Read the model definition and answer for the solid it produces. Units are mm, in the model's axes. Face numbers are marked on the shaded views. A direction names the side the tool comes from. Coordinates: 2 decimals unless noted, no trailing zeros. Write each loop counter-clockwise with the first axis right and the second up, starting at its lowest first coordinate (ties: lowest second). Pieces come first, ordered by that corner, then holes. Notation, with made-up numbers: M 69.5,-38 L 115.5,-38 A20 ccw 115.5,-24 Z; hole C 77,-37.75 d10. An arc over 180 degrees is marked long. Write item = value, one per line.
from build123d import *

# Parameters (mm, degrees)
BOSS_EXTRUDE1_DEPTH = 20
SKETCH7_R           = 70
CUT_EXTRUDE1_DEPTH  = 149.354929298


with BuildPart() as part:
    # Sketch4 → Boss-Extrude1 (new body)
    with BuildSketch(Plane.XY):
        Polygon((-50, -86.602540378), (50, -86.602540378), (100, 0), (50, 86.602540378), (-50, 86.602540378), (-100, 0), align=None)
        Polygon((-50, -86.602540378), (-110, 0), (-100, 0), align=None)
        Polygon((-100, 0), (-55, 95.262794416), (-50, 86.602540378), align=None)
        Polygon((-50, 86.602540378), (55, 95.262794416), (50, 86.602540378), align=None)
        Polygon((50, 86.602540378), (110, 0), (100, 0), align=None)
        Polygon((100, 0), (55, -95.262794416), (50, -86.602540378), align=None)
        Polygon((50, -86.602540378), (-55, -95.262794416), (-50, -86.602540378), align=None)
        with BuildLine():
            Line((-55, 95.262794416), (-50, 86.602540378))
            Line((-50, 86.602540378), (-50.900048654, 97.515050362))
            ThreePointArc((-50.900048654, 97.515050362), (-52.961998078, 96.410719111), (-55, 95.262794416))
        make_face()
        with BuildLine():
            Line((55, 95.262794416), (50, 86.602540378))
            Line((50, 86.602540378), (59.000486538, 92.838260369))
            ThreePointArc((59.000486538, 92.838260369), (57.013132909, 94.071795327), (55, 95.262794416))
        make_face()
        with BuildLine():
            Line((110, 0), (100, 0))
            Line((100, 0), (109.900535191, -4.676789993))
            ThreePointArc((109.900535191, -4.676789993), (109.975130987, -2.338923785), (110, 0))
        make_face()
        with BuildLine():
            Line((55, -95.262794416), (50, -86.602540378))
            Line((50, -86.602540378), (50.900048654, -97.515050362))
            ThreePointArc((50.900048654, -97.515050362), (52.961998078, -96.410719111), (55, -95.262794416))
        make_face()
        with BuildLine():
            Line((-55, -95.262794416), (-50, -86.602540378))
            Line((-50, -86.602540378), (-59.000486538, -92.838260369))
            ThreePointArc((-59.000486538, -92.838260369), (-57.013132909, -94.071795327), (-55, -95.262794416))
        make_face()
        with BuildLine():
            Line((-110, 0), (-100, 0))
            Line((-100, 0), (-109.900535191, 4.676789993))
            ThreePointArc((-109.900535191, 4.676789993), (-109.975130987, 2.338923785), (-110, 0))
        make_face()
    extrude(amount=BOSS_EXTRUDE1_DEPTH)

    # Sketch7 → Cut-Extrude1 (cut, through all)
    with BuildSketch(Plane(origin=(0, 0, 0), x_dir=(-1, 0, 0), z_dir=(0, 0, -1))):
        Circle(SKETCH7_R)
    extrude(amount=-CUT_EXTRUDE1_DEPTH, mode=Mode.SUBTRACT)


solid = part.part
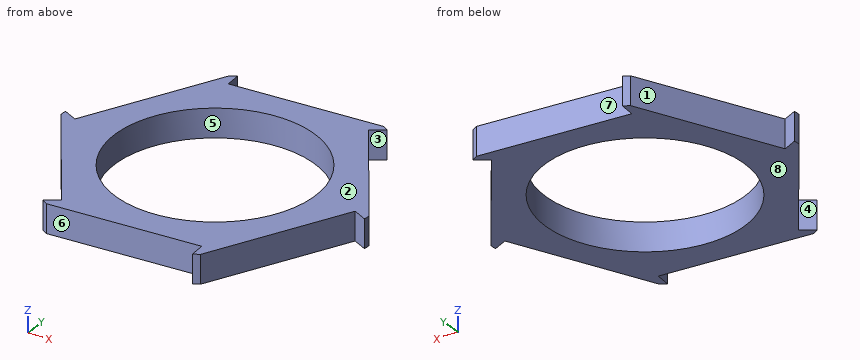
Item 1: Find section B-B (x = 0). Determine the outline of the cut face in (y, z).
Worked answers:
outline = M -90.73,0 L -70,0 L -70,20 L -90.73,20 Z; M 70,0 L 90.73,0 L 90.73,20 L 70,20 Z
Item 2: Consider line 1 along Y through (x, z) = (0, 14.5); line 2 along Y through (x, z) = (37.5, 2.5); line 3 along X through (y, z) = (6.5, 6). Determine where each line is inside the solid, lowest interval first. Write a range as from..to.
Worked answers:
line_1 = -90.73..-70, 70..90.73
line_2 = -87.63..-59.11, 59.11..93.82
line_3 = -96.93..-69.7, 69.7..105.5
Item 3: Find section A-A (z = 13.25). Determine the outline of the cut face in (x, y), and give its area (3 significant figures).
Worked answers:
outline = M -110,0 L -50,-86.6 L -59,-92.84 A110 ccw -55,-95.26 L 50,-86.6 L 50.9,-97.52 A110 ccw 55,-95.26 L 100,0 L 109.9,-4.68 A110 ccw 110,0 L 50,86.6 L 59,92.84 A110 ccw 55,95.26 L -50,86.6 L -50.9,97.52 A110 ccw -55,95.26 L -100,0 L -109.9,4.68 A110 ccw Z; hole C 0,0 d140
area = 13,300 mm²
Item 4: For a pull along Y with two mould halves and no side action, classify the marked faces 1, 2 and 3 as released by +Y, released by -Y, zero draft, split by the parting line, or undercut.
Worked answers:
face_1 = released by +Y
face_2 = zero draft
face_3 = undercut
Item 5: Find section C-C (y = -64). Determine the outline of the cut face in (x, z), and give its area (3 significant figures).
Worked answers:
outline = M -65.66,0 L -28.35,0 L -28.35,20 L -65.66,20 Z; M 28.35,0 L 69.77,0 L 69.77,20 L 28.35,20 Z
area = 1,570 mm²
Item 6: Which of the six approach directions +Z, -Z, +X, -X, +Y, -Y give full straight-line access (tool end or side, diameter ignored) to the marked faces 4, 5, 6, 7 and 8?
Worked answers:
face_4 = +Z, -Z, -X
face_5 = +Z, -Z
face_6 = +Z, -Z, -Y
face_7 = +Z, -Z, +Y
face_8 = -Z, +X, -X, +Y, -Y
Item 7: Find section D-D (x = -73). Determine the outline of the cut face in (y, z), and give its area (3 significant figures).
Worked answers:
outline = M -53.4,0 L 57.16,0 L 57.16,20 L -53.4,20 Z
area = 2,210 mm²
Item 8: Flat-ended cylindrical pins translate along their axes: pin 1 (5 mm diameter, centred on x = 87, z = 13.5, fed in from +Y); pin 2 (1.5 mm diameter, centred on x = -44.5, z = 16.5, fed in from +Y); pin 3 (8 mm diameter, centred on y = 27.5, z = 6.5, fed in from -X). Find the tip coordinate at first contact, or state that the pin passes through.
Worked answers:
pin_1 = 36.81
pin_2 = 87.12
pin_3 = -88.9
